Could you check a few things on this model? Use its own coordinates, in mm. A direction names the side the tool comes from. Coordinates: 2 decimals unless noted, no trailing zeros. Order: outer loops, then holes, each group sorted by start corner. A loop starts at its lowest first (then second) coordinate and runs counter-clockwise, first axis right, second up.
Solid Edge part; units mm, degrees
sketch "Sketch1" plane through (0.0007, 14.651, 5) normal (0, 0, 1) x (1, 0, 0)
  line L0 (-114.0407, 98.8093) -> (-57.2599, 131.5929)
  arc A0 (-54.1474, 131.5247) -> (-57.2599, 131.5929) centre (-55.7598, 128.9948) ccw
  arc A1 (-47.0142, 137.1861) -> (-48.7662, 134.4664) centre (-45.7662, 134.458) ccw
  arc A2 (-47.0142, 137.1861) -> (-26.9146, 142.5706) centre (-21.0226, 80.3698) cw
  arc A3 (-24.0376, 141.0909) -> (-26.9146, 142.5706) centre (-26.6317, 139.5839) ccw
  arc A4 (-15.245, 142.849) -> (-17.9063, 141.2336) centre (-15.245, 139.849) ccw
  line L1 (-15.245, 142.849) -> (15.2436, 142.849)
  arc A5 (17.905, 141.2336) -> (15.2436, 142.849) centre (15.2436, 139.849) ccw
  arc A6 (26.9132, 142.5696) -> (24.036, 141.0904) centre (26.6298, 139.583) ccw
  arc A7 (26.9132, 142.5696) -> (47.0027, 137.1869) centre (21.0099, 80.3561) cw
  arc A8 (48.7549, 134.4673) -> (47.0027, 137.1869) centre (45.7549, 134.4587) ccw
  arc A9 (57.2487, 131.5943) -> (54.1362, 131.526) centre (55.7487, 128.9962) ccw
  line L2 (57.2487, 131.5943) -> (114.0299, 98.8129)
  arc A10 (115.5271, 96.0833) -> (114.0299, 98.8129) centre (112.5299, 96.2148) ccw
  arc A11 (124.0003, 92.7805) -> (120.7849, 92.9052) centre (122.2944, 90.3127) ccw
  arc A12 (124.0003, 92.7805) -> (155.0355, 39.027) centre (82.7747, 33.1424) cw
  arc A13 (153.5358, 36.1799) -> (155.0355, 39.027) centre (152.0454, 38.7835) ccw
  arc A14 (155.2747, 27.3761) -> (153.6593, 30.0375) centre (152.2747, 27.3761) ccw
  line L3 (155.2747, 27.3761) -> (155.2747, -38.192)
  arc A15 (153.6593, -40.8534) -> (155.2747, -38.192) centre (152.2747, -38.192) ccw
  arc A16 (154.9954, -49.8615) -> (153.5161, -46.9844) centre (152.0088, -49.5782) ccw
  arc A17 (154.9954, -49.8615) -> (149.6134, -69.9554) centre (92.7533, -43.9583) cw
  arc A18 (146.8942, -71.7079) -> (149.6134, -69.9554) centre (146.8851, -68.7079) ccw
  arc A19 (144.0217, -80.2016) -> (143.9534, -77.0892) centre (141.4236, -78.7016) ccw
  line L4 (144.0217, -80.2016) -> (127.6444, -108.5679)
  arc A20 (122.7007, -116.5716) -> (122.8583, -113.3403) centre (120.256, -114.8329) ccw
  arc A21 (77.6703, -142.5696) -> (122.7007, -116.5716) centre (71.767, -80.3476) ccw
  arc A22 (74.7931, -141.0904) -> (77.6703, -142.5696) centre (77.3869, -139.583) ccw
  arc A23 (66.0007, -142.849) -> (68.6621, -141.2336) centre (66.0007, -139.849) ccw
  line L5 (5.7656, -142.849) -> (66.0007, -142.849)
  arc A24 (3.1042, -141.2336) -> (5.7656, -142.849) centre (5.7656, -139.849) ccw
  arc A25 (-5.767, -142.849) -> (-3.1056, -141.2336) centre (-5.767, -139.849) ccw
  line L6 (-66.0021, -142.849) -> (-5.767, -142.849)
  arc A26 (-68.6634, -141.2336) -> (-66.0021, -142.849) centre (-66.0021, -139.849) ccw
  arc A27 (-77.6716, -142.5694) -> (-74.7944, -141.0903) centre (-77.3881, -139.5828) ccw
  arc A28 (-122.6994, -116.5717) -> (-77.6716, -142.5694) centre (-71.7665, -80.349) ccw
  arc A29 (-122.857, -113.3404) -> (-122.6994, -116.5717) centre (-120.2547, -114.833) ccw
  arc A30 (-128.7762, -106.6053) -> (-126.0465, -108.1024) centre (-126.1781, -105.1053) ccw
  line L7 (-144.0218, -80.199) -> (-128.7762, -106.6053)
  arc A31 (-143.9535, -77.0865) -> (-144.0218, -80.199) centre (-141.4237, -78.699) ccw
  arc A32 (-149.6144, -69.9531) -> (-146.8949, -71.7053) centre (-146.8862, -68.7053) ccw
  arc A33 (-154.9987, -49.8585) -> (-149.6144, -69.9531) centre (-92.7672, -43.9523) ccw
  arc A34 (-153.5196, -46.9813) -> (-154.9987, -49.8585) centre (-152.0122, -49.5751) ccw
  arc A35 (-155.2786, -38.189) -> (-153.6631, -40.8503) centre (-152.2786, -38.1889) ccw
  line L8 (-155.2818, 27.3758) -> (-155.2786, -38.189)
  arc A36 (-153.6665, 30.0373) -> (-155.2818, 27.3758) centre (-152.2818, 27.376) ccw
  arc A37 (-155.0428, 39.0267) -> (-153.5432, 36.1796) centre (-152.0527, 38.7832) ccw
  arc A38 (-124.0109, 92.7765) -> (-155.0428, 39.0267) centre (-82.7847, 33.1421) ccw
  arc A39 (-120.7955, 92.9014) -> (-124.0109, 92.7765) centre (-122.3049, 90.3088) ccw
  arc A40 (-114.0407, 98.8093) -> (-115.5378, 96.0796) centre (-112.5406, 96.2112) ccw
  arc A41 (-48.7662, 134.4664) -> (-54.1474, 131.5247) centre (-52.2662, 134.4761) cw
  arc A42 (-17.9064, 141.2336) -> (-24.0377, 141.0909) centre (-21.0113, 142.849) cw
  arc A43 (24.036, 141.0904) -> (17.905, 141.2336) centre (21.0099, 142.849) cw
  arc A44 (54.1362, 131.526) -> (48.7549, 134.4673) centre (52.2549, 134.4774) cw
  arc A45 (120.7849, 92.9052) -> (115.5271, 96.0832) centre (119.0237, 95.9298) cw
  arc A46 (153.6593, 30.0375) -> (153.5358, 36.1799) centre (155.2747, 33.1424) cw
  arc A47 (153.5161, -46.9844) -> (153.6593, -40.8534) centre (155.2747, -43.9583) cw
  arc A48 (143.9534, -77.0891) -> (146.8942, -71.7079) centre (146.9048, -75.2079) cw
  arc A49 (122.8584, -113.3404) -> (127.6444, -108.5679) centre (125.8944, -111.599) cw
  arc A50 (68.6621, -141.2336) -> (74.7931, -141.0904) centre (71.767, -142.849) cw
  arc A51 (-3.1056, -141.2336) -> (3.1042, -141.2336) centre (-0.0007, -142.849) cw
  arc A52 (-74.7944, -141.0903) -> (-68.6635, -141.2336) centre (-71.7684, -142.849) cw
  arc A53 (-126.0466, -108.1024) -> (-122.857, -113.3404) centre (-125.8931, -111.599) cw
  arc A54 (-146.8949, -71.7053) -> (-143.9536, -77.0866) centre (-146.905, -75.2053) cw
  arc A55 (-153.6632, -40.8503) -> (-153.5196, -46.9813) centre (-155.2784, -43.9553) cw
  arc A56 (-153.5432, 36.1796) -> (-153.6665, 30.0373) centre (-155.2821, 33.1421) cw
  arc A57 (-115.5377, 96.0796) -> (-120.7955, 92.9014) centre (-119.0344, 95.926) cw
  line L9 (-56.0166, 140.971) -> (-122.7845, 102.4212)
  arc A58 (-162.7821, 33.1421) -> (-122.7845, 102.4212) centre (-82.7847, 33.1421) cw
  line L10 (-162.7821, 33.1421) -> (-162.7784, -43.9553)
  arc A59 (-162.7784, -43.9553) -> (-153.4002, -78.9553) centre (-92.7784, -43.9553) ccw
  line L11 (-132.3882, -115.349) -> (-153.4002, -78.9553)
  arc A60 (-132.3882, -115.349) -> (-71.7683, -150.349) centre (-71.7665, -80.349) ccw
  line L12 (71.767, -150.349) -> (-71.7683, -150.349)
  arc A61 (71.767, -150.349) -> (132.3896, -115.349) centre (71.7678, -80.349) ccw
  line L13 (132.3896, -115.349) -> (153.4002, -78.9576)
  arc A62 (162.7747, -43.9583) -> (153.4002, -78.9576) centre (92.791, -43.9684) cw
  line L14 (162.7747, 33.1424) -> (162.7747, -43.9583)
  arc A63 (122.7736, 102.4251) -> (162.7747, 33.1424) centre (82.7747, 33.1424) cw
  line L15 (56.0045, 140.9728) -> (122.7736, 102.4251)
  arc A64 (21.0099, 150.349) -> (56.0045, 140.9728) centre (21.008, 80.349) cw
  line L16 (-21.0112, 150.349) -> (21.0099, 150.349)
  arc A65 (-32.5074, 149.4015) -> (-21.0112, 150.349) centre (-20.997, 79.961) cw
  arc A66 (-44.641, 146.2432) -> (-32.5074, 149.4015) centre (-21.0122, 80.3518) cw
  arc A67 (-56.0166, 140.971) -> (-44.641, 146.2432) centre (-21.0122, 80.3518) cw
  circle A68 centre (-71.7683, -142.849) radius 1.5
  circle A69 centre (-0.0007, -142.849) radius 1.5
  circle A70 centre (-125.893, -111.599) radius 1.5
  circle A71 centre (-146.905, -75.2053) radius 1.5
  circle A72 centre (-155.2784, -43.9553) radius 1.5
  circle A73 centre (-155.2821, 33.1421) radius 1.5
  circle A74 centre (-119.0344, 95.9261) radius 1.5
  circle A75 centre (-52.2662, 134.4761) radius 1.5
  circle A76 centre (-21.0112, 142.849) radius 1.5
  circle A77 centre (21.0099, 142.849) radius 1.5
  circle A78 centre (52.2549, 134.4774) radius 1.5
  circle A79 centre (119.0237, 95.9298) radius 1.5
  circle A80 centre (155.2747, 33.1424) radius 1.5
  circle A81 centre (155.2747, -43.9583) radius 1.5
  circle A82 centre (146.9048, -75.2079) radius 1.5
  circle A83 centre (125.8944, -111.599) radius 1.5
  circle A84 centre (71.767, -142.849) radius 1.5
extrude "ExtrudedProtrusion_7" add sketch "Sketch1" along normal blind 5
sketch "Sketch2" plane through (-0.003, 14.651, 10) normal (0, 0, 1) x (1, 0, 0)
  line L0 (-170.0115, -5.4066) -> (169.0999, -5.4066)
  line L1 (169.0999, -5.4066) -> (169.0999, -159.984)
  line L2 (169.0999, -159.984) -> (-170.0115, -159.984)
  line L3 (-170.0115, -159.984) -> (-170.0115, -5.4066)
extrude "Cutout1" cut sketch "Sketch2" against normal up to next
properties material "Polycarbonate"
Item 1: Thinking about a two-plate mould opening in X: for faces 1 (the face through (-86.05, 129.62, 7.46)), 2 (the face through (-152.355, 87.282, 7.465)), 3 (the face through (-25, 157, 5)), which applies, +X half, -X half, draft (parallel to the pull), parting line (faces both ways), or undercut?
Item 2: Which directions (+Z, -Z, +X, -X, +Y, -Y) give clear straight access to the entire face, cutting with the end or side of a thin tool? Please do faces 4 (the face through (85.243, 130.084, 7.465)), 5 (the face through (-145.792, 83.652, 7.465)), 6 (the face through (88.92, 136.62, 7.46)).
Item 3: Suppose I cut it at A-A (y = 74.5). List the corners of the cut face in (x, z) for me, and give its area (3 significant figures).
Item 4: Suppose I cut it at D-D (x = 34.5). List the corners of the cut face in (y, z) for me, and give its area (3 significant figures).
Item 5: For pin 1 Ø5 at (x, y) = (119.02, 110.58) entering from +Z; pin 2 Ø1.5 at (y, z) = (140, 7.5) entering from -X; pin 3 Ø3 at (x, z) = (101.5, 6) entering from -Y; pin 4 Ø1.5 at (x, z) = (40, 9) entering from -Y, each with a flat end and sliding along its axis, tell me the tip position at first contact or that it passes through.
Item 6: Suppose I cut it at B-B (x = -83.5). List the corners of the cut face in (y, z) for me.
Item 7: Suppose I cut it at C-C (z = 6.4). Count the separate pieces of the cut face and the enclosed holes in it, and give its area (3 significant figures).
Item 8: I need wall thicknesses on line 1 (X direction, y = 35, z = 7.1); line 2 (Y direction, x = 52.5, z = 6.55); line 3 (X direction, y = 111.5, z = 8.8). Which ranges of each line are inside material? Lowest first, please.
Geometry results:
1. face 1: undercut
1. face 2: -X half
1. face 3: draft
2. face 4: +Z, -Z, -Y
2. face 5: +Z, -Z
2. face 6: +Z, -Z, +X, +Y
3. outline: (-158.19, 5) - (-150.18, 5) - (-150.18, 10) - (-158.19, 10) - close; (150.18, 5) - (158.19, 5) - (158.19, 10) - (150.18, 10) - close
3. area: 80.1 mm2
4. outline: (156.03, 5) - (163.69, 5) - (163.69, 10) - (156.03, 10) - close
4. area: 38.3 mm2
5. pin 1: stops at z = 10
5. pin 2: stops at x = -84.37
5. pin 3: stops at y = 119.83
5. pin 4: stops at y = 154.3
6. outline: (131.09, 5) - (139.75, 5) - (139.75, 10) - (131.09, 10) - close
7. separate pieces: 1
7. enclosed holes: 8
7. area: 3,880 mm2
8. line 1: x = -162.78 to -155.28, 155.28 to 162.78
8. line 2: y = 145.64 to 147.65, 150.61 to 157.52
8. line 3: x = -131.17 to -120.22, -117.85 to -115.47, 115.46 to 117.84, 120.21 to 131.16
